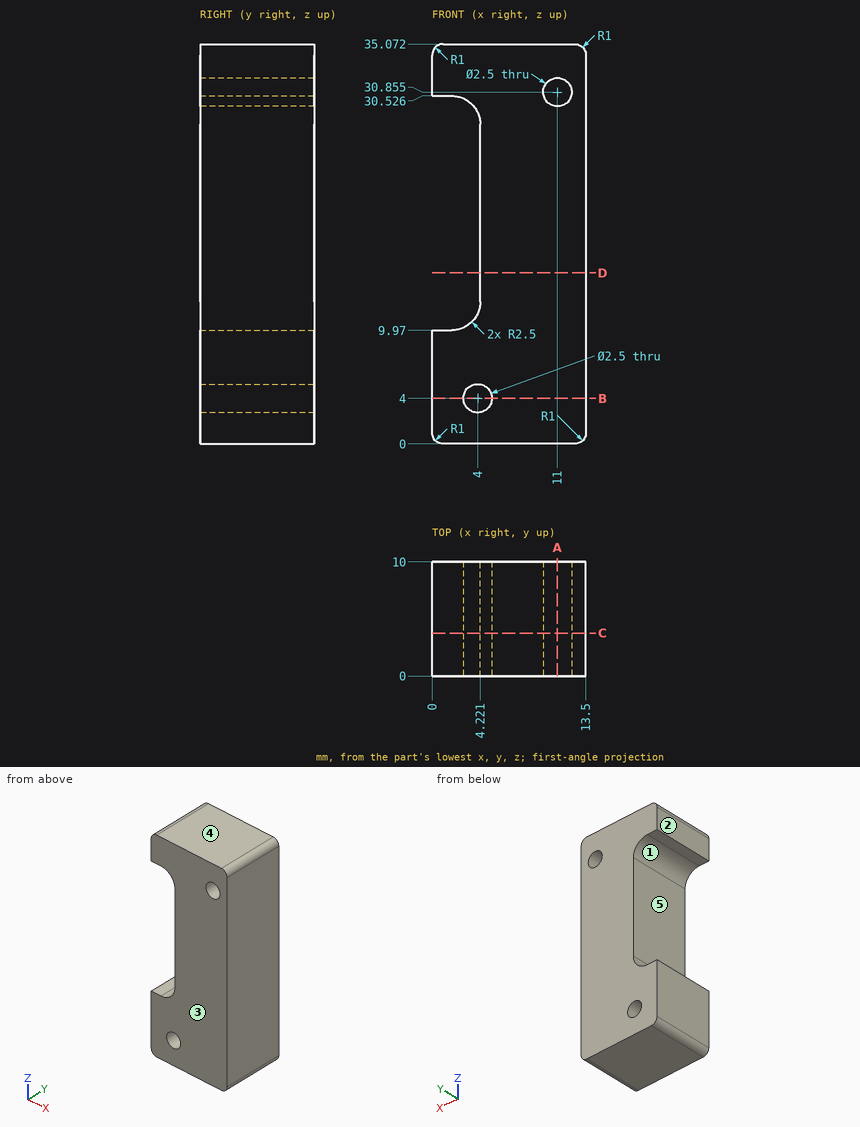
Input: dimensioned drawing with shaded views. Units: mm. Origin: part minimum x, y, z. A direction names the side the tool comes from. Coordinates: 2 decimals unless noted, no trailing zeros. Loops run counter-clockwise (first coordinate to the right, second up) from the corner with the lowest first, then second, coordinate; pieces in that order, holes last. Notation, with made-up numbers: M 68.25,-14 L 118.25,-14 A20 ccw 118.25,-10 Z; hole C 48.5,-16.5 d3. An arc over 180 degrees is marked long. Use a Markdown table: item, result. Add a question column.
Q1. Access query for the marked faces 1 and 2. Directions: +Z, -Z, +X, -X, +Y, -Y. A direction counts if a zero-diameter tool reaches every point of the face in a straight line with its end or side. Return the directions, or none.
Q2. Section query C-C, the plane y = 3.75. State how many separate pieces and enclosed holes the cut face has, and give its area (3 significant figures).
Q3. Section query D-D, the plane z = 15. Return loops of the section in (x, y), and give its area (3 significant figures).
Q4. Section query A-A, the plane x = 11. Return loops of the section in (y, z) (1 decimal), and give its area (3 significant figures).
Q5. Draft query along Z for the marked faces 3, 4 and 5. Return one class per face: pulls with the +Z half, pulls with the -Z half, needs draft (parallel to the pull), parting line crosses it, or undercut.
Q6. Material intervals for L1, parallel to X at y = 5.25, z = 4; L2, parallel to Z at x = 1.75, y = 5.5; L3, parallel to Z at x = 3.5, y = 5.75 (1 decimal), sorted ascending.
Q7. Section query B-B, the plane z = 4. Return loops of the section in (x, y), and give its area (3 significant figures).
Result:
| question | item | result |
|---|---|---|
| 1 | face 1 | -X, +Y, -Y |
| 1 | face 2 | +Z, -Z, -X, +Y, -Y |
| 2 | separate pieces | 1 |
| 2 | enclosed holes | 2 |
| 2 | area | 379 mm2 |
| 3 | outline | M 4.22,0 L 13.5,0 L 13.5,10 L 4.22,10 Z |
| 3 | area | 92.8 mm2 |
| 4 | outline | M 0,0 L 10,0 L 10,29.6 L 0,29.6 Z; M 0,32.1 L 10,32.1 L 10,35.1 L 0,35.1 Z |
| 4 | area | 326 mm2 |
| 5 | face 3 | needs draft |
| 5 | face 4 | pulls with the +Z half |
| 5 | face 5 | undercut |
| 6 | L1 | x = 0 to 2.75, 5.25 to 13.5 |
| 6 | L2 | z = 0 to 9.97, 30.53 to 35.07 |
| 6 | L3 | z = 0 to 2.9, 5.1 to 10.7, 29.8 to 35.1 |
| 7 | outline | M 0,0 L 2.75,0 L 2.75,10 L 0,10 Z; M 5.25,0 L 13.5,0 L 13.5,10 L 5.25,10 Z |
| 7 | area | 110 mm2 |
